from build123d import *

# Parameters (mm, degrees)
F2_R = 1


with BuildPart() as f1:
    # F0 (on Front) → F1 (revolve)
    with BuildSketch(Plane.XZ):
        Polygon((29.0886, 52.241075), (8.428346, 52.241075), (8.428346, 23.81056), (17.0886, 18.81056), (29.0886, 18.81056), align=None)
    revolve(axis=Axis((0, 0, 34.322324), (0, 0, 1)))

    # F2
    f2_edges = [f1.edges().sort_by_distance(p)[0] for p in [
        (-29.0886, 0, 52.241075),
        (-8.428346, 0, 52.241075),
    ]]
    fillet(f2_edges, radius=F2_R)


solid = f1.part
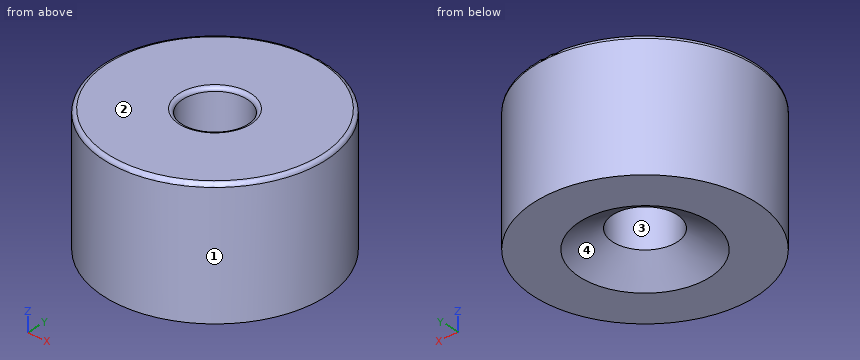
Geometry check sheet. Reference: the model listing, model coordinates, mm. Face numbers are marked on the shaded views. Give positions to 0.01 mm unless a question says otherwise; leave off trailing zeros. Loops run counter-clockwise (first coordinate to the right, second up) from the corner with the lowest first, then second, coordinate; pieces in that order, holes last. Notation, with made-up numbers: (42.5, 2) -> (97.5, 2) arc R11 cw to (97.5, 22) -> close; hole circle Ø11 at (4, 34). An arc over 180 degrees is marked (long way). Answer in a Markdown table with one row per item. Add a question column.
1) Material ranges on probe 1 along Y at (x, z) = (0, 34.75); probe 2 along Y at (x, z) = (2, 23.5); probe 3 along Y at (x, z) = (-17.5, 50.5), recorded low to high. Write a range as from..to.
2) Gauge pin test, flat ends, axial feed: P1, Ø3, axis at x = 5, z = 40, coming from the +Y side; P2, Ø5, axis at x = -6.5, y = 1, coming from the -Z side; P3, Ø1.5, axis at y = -21, z = 34.5, coming from the -X side. Record the tip position at first contact, or that the pin passes through.
3) Cross-section at A-A on y = 0. Record the boundary of the cut face in (x, z), and give its area (3 significant figures).
4) Cross-section at C-C on z = 32. Record the boundary of the cut face in (x, y), and give its area (3 significant figures).
5) Draft check along Y on the marked faces 1, 2, 3 and 4. Enter one of: pulls with the +Y half, pulls with the -Y half, needs draft (parallel to the pull), parting line crosses it, or undercut.
Outcome:
| question | item | result |
|---|---|---|
| 1 | probe 1 | y = -29.09..-8.43, 8.43..29.09 |
| 1 | probe 2 | y = -29.02..-8.74, 8.74..29.02 |
| 1 | probe 3 | y = -23.24..23.24 |
| 2 | P1 | stops at y = 28.88 |
| 2 | P2 | stops at z = 23.44 |
| 2 | P3 | stops at x = -20.88 |
| 3 | outline | (-29.09, 18.81) -> (-17.09, 18.81) -> (-8.43, 23.81) -> (-8.43, 51.24) arc R1 ccw to (-9.43, 52.24) -> (-28.09, 52.24) arc R1 ccw to (-29.09, 51.24) -> close; (8.43, 23.81) -> (17.09, 18.81) -> (29.09, 18.81) -> (29.09, 51.24) arc R1 ccw to (28.09, 52.24) -> (9.43, 52.24) arc R1 ccw to (8.43, 51.24) -> close |
| 3 | area | 1,340 mm^2 |
| 4 | outline | circle Ø58.18 at (0, 0); hole circle Ø16.86 at (0, 0) |
| 4 | area | 2,440 mm^2 |
| 5 | face 1 | parting line crosses it |
| 5 | face 2 | needs draft |
| 5 | face 3 | undercut |
| 5 | face 4 | undercut |
